from build123d import *

# Parameters (mm, degrees)
SKETCH2_W            = 19
SKETCH2_H            = 0.15
M3_CLEARANCE_HOLE1_D = 3.2
CUT_EXTRUDE1_REACH   = 181.373
SKETCH5_R            = 1.6
MOVE_FACE1_BY        = 15
MOVE_FACE1_2_BY      = 15
FILLET1_R            = 9.5


with BuildPart() as part:
    # Sweep1: sweep along a path in tape_measure_path
    with BuildLine(Plane.XY) as sweep1_path:
        Line((0, 0), (18, 0))
        ThreePointArc((18, 0), (21.535533906, -1.464466094), (23, -5))
        Line((23, -5), (23, -106.544934808))
        ThreePointArc((23, -106.544934808), (63, -146.544934808), (103, -106.544934808))
        Line((103, -106.544934808), (103, -9.607557393))
    # Sketch2 → Sweep1 (sweep)
    with BuildSketch(Plane(origin=(0, 0, 0), x_dir=(0, 0, -1), z_dir=(1, 0, 0))):
        with Locations((0, 0.075)):
            Rectangle(SKETCH2_W, SKETCH2_H)
    sweep(path=sweep1_path.line)

    # M3 Clearance Hole1 (through all)
    with Locations(Plane(origin=(0, 0.15, 0), x_dir=(1, 0, 0), z_dir=(0, 1, 0))):
        with Locations((4, 0), (14, 0)):
            Hole(M3_CLEARANCE_HOLE1_D / 2)

    # Sketch5 → Cut-Extrude1 (cut, up to next)
    with BuildSketch(Plane(origin=(103, 0, 0), x_dir=(0, 0, -1), z_dir=(1, 0, 0)), mode=Mode.PRIVATE) as cut_extrude1_sk1:
        with Locations(Location((0, -13.607557393, 0), (0, 0, 90))):
            Circle(SKETCH5_R)
    cut_extrude1_tool1 = extrude(cut_extrude1_sk1.sketch, amount=-CUT_EXTRUDE1_REACH, mode=Mode.PRIVATE) & part.part
    # Sketch5 → Cut-Extrude1 (cut, up to next)
    with BuildSketch(Plane(origin=(103, 0, 0), x_dir=(0, 0, -1), z_dir=(1, 0, 0)), mode=Mode.PRIVATE) as cut_extrude1_sk2:
        with Locations(Location((0, -23.607557393, 0), (0, 0, 90))):
            Circle(SKETCH5_R)
    cut_extrude1_tool2 = extrude(cut_extrude1_sk2.sketch, amount=-CUT_EXTRUDE1_REACH, mode=Mode.PRIVATE) & part.part
    add(cut_extrude1_tool1.solids().sort_by_distance((103, -13.607557, 0))[0], mode=Mode.SUBTRACT)
    add(cut_extrude1_tool2.solids().sort_by_distance((103, -23.607557, 0))[0], mode=Mode.SUBTRACT)

    # Move Face1: a face moved outward by 15.0
    extrude(part.faces().sort_by_distance((102.925, -9.607557393, 0))[0], amount=MOVE_FACE1_BY, dir=(0, 1, 0))

    # Move Face1 2: a face moved outward by 15.0
    extrude(part.faces().sort_by_distance((0, 0.075, 0))[0], amount=MOVE_FACE1_2_BY, dir=(-1, 0, 0))

    # Fillet1
    fillet1_edges = [part.edges().sort_by_distance(p)[0] for p in [
        (-15, 0.075, 9.5),
        (-15, 0.075, -9.5),
        (102.925, 5.392442607, 9.5),
        (102.925, 5.392442607, -9.5),
    ]]
    fillet(fillet1_edges, radius=FILLET1_R - 0.0001)  # a hair under: the kernel refuses the full size


solid = part.part
Work out the finished part from the listing and answer in its coordinate system (mm). Coordinates: 2 decimals unless noted, no trailing zeros. Write each loop counter-clockwise with the first axis right and the second up, starting at its lowest first coordinate (ties: lowest second). Pieces come first, ordered by that corner, then holes. Notation, with made-up numbers: M 33.25,-11 L 62.25,-11 A8 ccw 62.25,-6 Z; hole C 36.25,-19.75 d3. An arc over 180 degrees is marked long. Answer as CSV lines item,"result". Start each with the question number.
Item 1: Flat-ended cylindrical pins translate along their axes: P1, Ø4, axis at x = 14, z = 0, coming from the +Y side; P2, Ø3, axis at y = -101, z = 0.5, coming from the -X side; P3, Ø3.5, axis at y = -13.61, z = 0, coming from the +X side; P4, Ø3, axis at x = 21, z = 3, coming from the +Y side. Find the tip coordinate at first contact, or state that the pin passes through.
Item 2: Section D-D on x = 63 is taken. Write down the section's boundary in (y, z), and give its area (3 significant figures).
Item 3: Section B-B on x = 4 is taken. Write down the section's boundary in (y, z), and give its area (3 significant figures).
Item 4: Consider L1, parallel to Z at x = 4, y = 0.1; L2, parallel to Y at x = 12, z = -7.5; L3, parallel to Y at x = 82, z = 6.75. Determine where each line is inside the solid, lowest interval first.
Item 5: Section C-C on z = 6.5 is taken. Write down the section's boundary in (x, y).
Item 6: Determine the mould class of faces 1 (the face through (62.124, -146.385, 0.133)), 2 (the face through (21, -1, 0)), 3 (the face through (103, -51, 0)) for opening direction X: released by +X, released by -X, zero draft, split by the parting line, or undercut.
Item 7: Section A-A on y = -28 is taken. Write down the section's boundary in (x, z), and give its area (3 significant figures).
Checks:
1,P1,"stops at y = 0.15"
1,P2,"stops at x = 23"
1,P3,"stops at x = 103"
1,P4,"stops at y = -0.07"
2,outline,"M -146.54,-9.5 L -146.39,-9.5 L -146.39,9.5 L -146.54,9.5 Z"
2,area,"2.85 mm²"
3,outline,"M 0,-9.5 L 0.15,-9.5 L 0.15,-1.6 L 0,-1.6 Z; M 0,1.6 L 0.15,1.6 L 0.15,9.5 L 0,9.5 Z"
3,area,"2.37 mm²"
4,L1,"z = -9.5 to -1.6, 1.6 to 9.5"
4,L2,"y = 0 to 0.15"
4,L3,"y = -141.74 to -141.57"
5,outline,"M -12.43,0 L 18,0 A5 cw 23,-5 L 23,-106.54 A40 ccw 103,-106.54 L 103,2.82 L 102.85,2.82 L 102.85,-106.54 A39.85 cw 23.15,-106.54 L 23.15,-5 A5.15 ccw 18,0.15 L -12.43,0.15 Z"
6,face 1,"undercut"
6,face 2,"released by -X"
6,face 3,"released by +X"
7,outline,"M 23,-9.5 L 23.15,-9.5 L 23.15,9.5 L 23,9.5 Z; M 102.85,-9.5 L 103,-9.5 L 103,9.5 L 102.85,9.5 Z"
7,area,"5.70 mm²"
